Geometry: final body of the model. Coordinates: model frame, mm. Round coordinates to 2 decimals unless told otherwise and drop trailing zeros. Order: outer loops, then holes, each group sorted by start corner. A loop starts at its lowest first (then second) coordinate and runs counter-clockwise, first axis right, second up. Notation, with made-up numbers: (73, 42) - (86, 42) arc R23 ccw to (86, 58) - close; hole circle Ø7 at (89.25, 63). An arc over 180 degrees is marked (long way). Put each result on its own line as item: value. Start each with the question number.
(1) Section A-A (z = 0). Output: boundary loops of the cut face in (x, y).
(2) Section C-C (y = -19.5). Output: boundary loops of the cut face in (x, z), and give its area (3 significant figures).
(3) Pin query (flat end, axial travel): P1, Ø6, axis at x = 2, y = -29.5, coming from the +Z side; P2, Ø3, axis at x = 7, z = -33, coming from the -Y side; P3, Ø1.5, axis at x = 1.5, z = -37, coming from the +Y side; P4, Ø20, axis at y = 0, z = 0, coming from the -X side. Return the tip coordinate at first contact, or that it passes through.
(4) Material intervals for L1, parallel to Y at x = 4.25, z = 0; L2, parallel to Y at x = 1.5, z = 27.5; L3, parallel to Z at x = 6, y = -16, sorted ascending. Write a range as [from, to].
(5) Pull-direction query (Y, two-part tool) for faces 1 (the face through (4.93, -16.49, -16.39)), 2 (the face through (10, -10, -10)); classes: released by +Y, released by -Y, zero draft, split by the parting line, or undercut.
(6) Section B-B (x = 8.5). Count the separate pieces of the cut face and the enclosed holes in it, and give its area (3 significant figures).
(7) Section D-D (y = 30). Output: boundary loops of the cut face in (x, z), and give its area (3 significant figures).
from build123d import *

# Parameters (mm, degrees)
SKETCH1_R             = 50
BOSS_EXTRUDE2_DEPTH   = 10
SKETCH1_4_OUTSIDE_W   = 130.354
SKETCH1_4_OUTSIDE_H   = 130.354
SKETCH1_4_OUTSIDE_R   = 50
SKETCH1_4_OUTSIDE_R_2 = 12.5
CUT_EXTRUDE2_DEPTH    = 13


with BuildPart() as part:
    # Sketch1 → Boss-Extrude2 (new body)
    with BuildSketch(Plane(origin=(0, 0, 0), x_dir=(0, 0, -1), z_dir=(1, 0, 0))):
        Circle(SKETCH1_R)
    extrude(amount=BOSS_EXTRUDE2_DEPTH)

    # Sketch1_4 outside → Cut-Extrude2 (cut)
    # profile 1 of 10: a face of its own
    with BuildSketch(Plane(origin=(0, 0, 0), x_dir=(0, 0, -1), z_dir=(1, 0, 0))):
        Rectangle(SKETCH1_4_OUTSIDE_W, SKETCH1_4_OUTSIDE_H)
        Circle(SKETCH1_4_OUTSIDE_R, mode=Mode.SUBTRACT)
    # profile 2 of 10: a face of its own
    with BuildSketch(Plane(origin=(0, 0, 0), x_dir=(0, 0, -1), z_dir=(1, 0, 0))):
        with Locations(Location((0, 0, 0), (0, 0, 180))):
            Circle(SKETCH1_4_OUTSIDE_R_2)
    # profile 3 of 10: a face of its own
    with BuildSketch(Plane(origin=(0, 0, 0), x_dir=(0, 0, -1), z_dir=(1, 0, 0))):
        with BuildLine():
            Line((3, 36.25), (3, 26.25))
            ThreePointArc((3, 26.25), (0, 23.25), (-3, 26.25))
            Line((-3, 26.25), (-3, 36.25))
            ThreePointArc((-3, 36.25), (0, 39.25), (3, 36.25))
        make_face()
    # profile 4 of 10: a face of its own
    with BuildSketch(Plane(origin=(0, 0, 0), x_dir=(0, 0, -1), z_dir=(1, 0, 0))):
        with BuildLine():
            Line((27.753941162, 23.511300474), (20.68287335, 16.440232663))
            ThreePointArc((20.68287335, 16.440232663), (16.440232663, 16.440232663), (16.440232663, 20.68287335))
            Line((16.440232663, 20.68287335), (23.511300474, 27.753941162))
            ThreePointArc((23.511300474, 27.753941162), (27.753941162, 27.753941162), (27.753941162, 23.511300474))
        make_face()
    # profile 5 of 10: a face of its own
    with BuildSketch(Plane(origin=(0, 0, 0), x_dir=(0, 0, -1), z_dir=(1, 0, 0))):
        with BuildLine():
            Line((36.25, -3), (26.25, -3))
            ThreePointArc((26.25, -3), (23.25, 0), (26.25, 3))
            Line((26.25, 3), (36.25, 3))
            ThreePointArc((36.25, 3), (39.25, 0), (36.25, -3))
        make_face()
    # profile 6 of 10: a face of its own
    with BuildSketch(Plane(origin=(0, 0, 0), x_dir=(0, 0, -1), z_dir=(1, 0, 0))):
        with BuildLine():
            Line((23.511300474, -27.753941162), (16.440232663, -20.68287335))
            ThreePointArc((16.440232663, -20.68287335), (16.440232663, -16.440232663), (20.68287335, -16.440232663))
            Line((20.68287335, -16.440232663), (27.753941162, -23.511300474))
            ThreePointArc((27.753941162, -23.511300474), (27.753941162, -27.753941162), (23.511300474, -27.753941162))
        make_face()
    # profile 7 of 10: a face of its own
    with BuildSketch(Plane(origin=(0, 0, 0), x_dir=(0, 0, -1), z_dir=(1, 0, 0))):
        with BuildLine():
            Line((-3, -36.25), (-3, -26.25))
            ThreePointArc((-3, -26.25), (0, -23.25), (3, -26.25))
            Line((3, -26.25), (3, -36.25))
            ThreePointArc((3, -36.25), (0, -39.25), (-3, -36.25))
        make_face()
    # profile 8 of 10: a face of its own
    with BuildSketch(Plane(origin=(0, 0, 0), x_dir=(0, 0, -1), z_dir=(1, 0, 0))):
        with BuildLine():
            Line((-27.753941162, -23.511300474), (-20.68287335, -16.440232663))
            ThreePointArc((-20.68287335, -16.440232663), (-16.440232663, -16.440232663), (-16.440232663, -20.68287335))
            Line((-16.440232663, -20.68287335), (-23.511300474, -27.753941162))
            ThreePointArc((-23.511300474, -27.753941162), (-27.753941162, -27.753941162), (-27.753941162, -23.511300474))
        make_face()
    # profile 9 of 10: a face of its own
    with BuildSketch(Plane(origin=(0, 0, 0), x_dir=(0, 0, -1), z_dir=(1, 0, 0))):
        with BuildLine():
            Line((-36.25, 3), (-26.25, 3))
            ThreePointArc((-26.25, 3), (-23.25, 0), (-26.25, -3))
            Line((-26.25, -3), (-36.25, -3))
            ThreePointArc((-36.25, -3), (-39.25, 0), (-36.25, 3))
        make_face()
    # profile 10 of 10: a face of its own
    with BuildSketch(Plane(origin=(0, 0, 0), x_dir=(0, 0, -1), z_dir=(1, 0, 0))):
        with BuildLine():
            Line((-23.511300474, 27.753941162), (-16.440232663, 20.68287335))
            ThreePointArc((-16.440232663, 20.68287335), (-16.440232663, 16.440232663), (-20.68287335, 16.440232663))
            Line((-20.68287335, 16.440232663), (-27.753941162, 23.511300474))
            ThreePointArc((-27.753941162, 23.511300474), (-27.753941162, 27.753941162), (-23.511300474, 27.753941162))
        make_face()
    extrude(amount=CUT_EXTRUDE2_DEPTH, mode=Mode.SUBTRACT)


solid = part.part
Checks:
1. outline: (0, -50) - (10, -50) - (10, -39.25) - (0, -39.25) - close; (0, -23.25) - (10, -23.25) - (10, -12.5) - (0, -12.5) - close; (0, 12.5) - (10, 12.5) - (10, 23.25) - (0, 23.25) - close; (0, 39.25) - (10, 39.25) - (10, 50) - (0, 50) - close
2. outline: (0, -46.04) - (10, -46.04) - (10, -23.74) - (0, -23.74) - close; (0, -15.71) - (10, -15.71) - (10, 15.71) - (0, 15.71) - close; (0, 23.74) - (10, 23.74) - (10, 46.04) - (0, 46.04) - close
2. area: 760 mm²
3. P1: stops at z = 42.4
3. P2: stops at y = -38.83
3. P3: stops at y = 34.44
3. P4: passes through
4. L1: y = [-50, -39.25], [-23.25, -12.5], [12.5, 23.25], [39.25, 50]
4. L2: y = [-41.76, -27.98], [-23.26, -3], [3, 23.26], [27.98, 41.76]
4. L3: z = [-47.37, -20.12], [-17, 17], [20.12, 47.37]
5. face 1: undercut
5. face 2: zero draft
6. separate pieces: 1
6. enclosed holes: 9
6. area: 6,660 mm²
7. outline: (0, -40) - (10, -40) - (10, -3) - (0, -3) - close; (0, 3) - (10, 3) - (10, 40) - (0, 40) - close
7. area: 740 mm²
